Part model, mm, in its own coordinate system. A direction names the side the tool comes from. Round coordinates to 2 decimals unless told otherwise and drop trailing zeros. Write each loop counter-clockwise with the first axis right and the second up, starting at its lowest first coordinate (ties: lowest second). Pieces come first, ordered by that corner, then holes.
Autodesk Inventor part; units mm, degrees
ref_plane "YZ Plane" through (0, 0, 0) normal (1, 0, 0) x (0, 1, 0)
ref_plane "XZ Plane" through (0, 0, 0) normal (0, 1, 0) x (-1, 0, 0)
ref_plane "XY Plane" through (0, 0, 0) normal (0, 0, 1) x (1, 0, 0)
sketch "Szkic1" plane through (0, 0, 0) normal (0, 0, 1) x (1, 0, 0)
  line L0 (-10.3866, 5.557) -> (25.6134, 5.557)
  line L1 (25.6134, 5.557) -> (25.6134, -36.443)
  line L2 (25.6134, -36.443) -> (-10.3866, -36.443)
  line L3 (-10.3866, -36.443) -> (-10.3866, 5.557)
  point P0 (0, 0)
  point P1 (20.6134, -0.193)
  point P2 (20.6134, -30.693)
  point P3 (-5.3866, -0.193)
  point P4 (-5.3866, -30.693)
  dimension "d0" = 36
  dimension "d1" = 42
  dimension "d2" = 5
  dimension "d3" = 5
  dimension "d4" = 5
  dimension "d5" = 5
  dimension "d6" = 5.75
  dimension "d7" = 5.75
  dimension "d8" = 5.75
  dimension "d9" = 5.75
extrude "Wyciągnięcie proste1" add sketch "Szkic1" along normal blind 7.5
hole "Otwór1" at (20.6134, -0.193, 0) at (20.6134, -30.693, 0) at (-5.3866, -0.193, 0) at (-5.3866, -30.693, 0) direction (0, 0, 1) diameter 5 end through all
sketch "Szkic2" plane through (-10.3866, -36.443, 0) normal (0, -1, 0) x (1, 0, 0)
  line L0 (36, 0) -> (0, 0)
  line L1 (36, 0) -> (36, 7.5)
  line L2 (0, 7.5) -> (36, 7.5)
  line L3 (0, 0) -> (0, 7.5)
  line L4 (36, 7.5) -> (0, 7.5)
  circle A0 centre (18, 8.5) radius 5.05
  point P0 (10.3866, 0)
  dimension "d19" = 36
  dimension "d25" = 8.5
  dimension "d26" = 18
  dimension "d27" = 10.1
extrude "Wyciągnięcie proste2" cut sketch "Szkic2" against normal through all contours A0 L2 | L2 A0
sketch "Szkic3" plane through (0, 0, 7.5) normal (0, 0, 1) x (1, 0, 0)
  line L0 (25.6134, 5.557) -> (12.5634, 5.557)
  line L1 (12.5634, 5.557) -> (12.5634, -36.443)
  line L2 (-10.3866, -36.443) -> (2.6634, -36.443)
  line L3 (25.6134, -36.443) -> (25.6134, 5.557)
  circle A0 centre (20.6134, -0.193) radius 2.5
  circle A1 centre (20.6134, -30.693) radius 2.5
  line L4 (12.5634, -36.443) -> (25.6134, -36.443)
  line L5 (2.6634, -36.443) -> (2.6634, 5.557)
  line L6 (2.6634, 5.557) -> (-10.3866, 5.557)
  line L7 (-10.3866, 5.557) -> (-10.3866, -36.443)
  point P0 (0, 0)
extrude "Wyciągnięcie proste3" add sketch "Szkic3" along normal blind 1 contours L3 L4 L1 L0
sketch "Szkic4" plane through (0, 0, 0) normal (0, 0, -1) x (-1, 0, 0)
  circle A0 centre (5.3866, -0.193) radius 2.5
  circle A1 centre (-20.6134, -0.193) radius 2.5
  circle A2 centre (-20.6134, -30.693) radius 2.5
  circle A3 centre (5.3866, -30.693) radius 2.5
  line L0 (10.3866, 5.557) -> (-25.6134, 5.557)
  line L1 (-25.6134, 5.557) -> (-25.6134, -36.443)
  line L2 (-25.6134, -36.443) -> (10.3866, -36.443)
  line L3 (10.3866, -36.443) -> (10.3866, 5.557)
  line L4 (-25.6134, 5.557) -> (-25.6134, 23.557)
  line L5 (-25.6134, 23.557) -> (-19.6134, 23.557)
  line L6 (-19.6134, 23.557) -> (-19.6134, 5.557)
  point P0 (0, 0)
  dimension "d30" = 18
  dimension "d31" = 6
extrude "Wyciągnięcie proste4" add sketch "Szkic4" against normal blind 8.5 contours L0 L4 L5 L6
sketch "Szkic5" plane through (19.6134, 5.557, 0) normal (-1, 0, 0) x (0, 0, 1)
  line L0 (0, 0) -> (0, 18)
  line L1 (8.5, 0) -> (0, 0)
  line L2 (8.5, 18) -> (8.5, 0)
  line L3 (0, 18) -> (8.5, 18)
  point P0 (0, -5.557)
  point P1 (4.25, 14)
  dimension "d34" = 4.25
  dimension "d35" = 4
  dimension "d47" = 8.5
hole "Otwór2" at (19.6134, 19.557, 4.25) direction (1, 0, 0) diameter 3 end through all
chamfer "Faza1" distance 3 angle 45 1 edges at (19.6134, 5.557, 4.25)
fillet "Zaokrąglenie2" radius 1 5 edges at (-10.3866, 5.557, 3.75) (-10.3866, -36.443, 3.75) (25.6134, -36.443, 4.25) (19.6134, 8.557, 4.25) (16.6134, 5.557, 4.25)
sketch "Szkic6" plane through (7.6134, -36.443, 8.5) normal (0, -1, 0) x (1, 0, 0)
  line L0 (17, 0) -> (17, -8.5)
  line L1 (4.95, 0) -> (17, 0)
  line L2 (4.95, -1) -> (4.95, 0)
  arc A0 (-4.95, -1) -> (4.95, -1) centre (0, 0) ccw
  line L3 (-17, -1) -> (-4.95, -1)
  line L4 (-17, -8.5) -> (-17, -1)
  line L5 (17, -8.5) -> (-17, -8.5)
  circle A1 centre (0, 0) radius 5.05
  point P0 (-7.6134, -8.5)
  dimension "d49" = 10.1
extrude "Wyciągnięcie proste5" cut sketch "Szkic6" against normal through all contours A1 L2 L1 | L1 L2 A0 A1
fillet "Zaokrąglenie3" radius 0.5 2 edges at (19.6134, 23.557, 4.25) (25.6134, 23.557, 4.25)
properties part number "3DP_ABS_X_Axis_Linear_Shaft_Clamp_Bottom_With_Endstop_Screw"
Q1. Cut at B-B on y = -29.5. Write the cut outline in (x, z).
Values follow:
outline: (-10.39, 0) - (-7.58, 0) - (-7.58, 7.5) - (-10.39, 7.5) - close; (-3.19, 0) - (18.42, 0) - (18.42, 8.5) - (12.66, 8.5) arc R5.05 cw to (2.66, 7.5) - (-3.19, 7.5) - close; (22.81, 0) - (25.61, 0) - (25.61, 8.5) - (22.81, 8.5) - close
Q2. Drop flat-ended pins along their axis: pin 1 (2.5 mm diameter, centred on y = 14.5, z = 3.5, fed in from -X); pin 2 (4 mm diameter, centred on x = 2, z = 6, fed in from +Y); pin 3 (6.5 mm diameter, centred on x = -4.5, y = -8.5, fed in from +Z). Give the stop position or say it passes through.
Values follow:
pin 1: stops at x = 19.61
pin 2: stops at y = 5.56
pin 3: stops at z = 7.5
Q3. Cut at D-D on z = 1. Write the cut outline in (x, y).
Values follow:
outline: (-10.39, -35.44) arc R1 ccw to (-9.39, -36.44) - (24.61, -36.44) arc R1 ccw to (25.61, -35.44) - (25.61, 23.06) arc R0.5 ccw to (25.11, 23.56) - (20.11, 23.56) arc R0.5 ccw to (19.61, 23.06) - (19.61, 8.97) arc R1 cw to (19.32, 8.26) - (16.91, 5.85) arc R1 cw to (16.2, 5.56) - (-9.39, 5.56) arc R1 ccw to (-10.39, 4.56) - close; hole circle Ø5 at (-5.39, -30.69); hole circle Ø5 at (-5.39, -0.19); hole circle Ø5 at (20.61, -30.69); hole circle Ø5 at (20.61, -0.19)
Q4. Cut at C-C on x = -7. Write the cut outline in (y, z).
Values follow:
outline: (-36.44, 0) - (-32.6, 0) - (-32.6, 7.5) - (-36.44, 7.5) - close; (-28.78, 0) - (-2.1, 0) - (-2.1, 7.5) - (-28.78, 7.5) - close; (1.72, 0) - (5.56, 0) - (5.56, 7.5) - (1.72, 7.5) - close
Q5. Mould opens along X. For faces 3 (the cylindrical face through (-3.87, -32.68, 3.8)), 4 (the flat face through (-4, -15, 7.5)), 5 (the flat face through (18.097, 7.04, 4.19)) say: +X half, -X half, draft (parallel to the pull), parting line (faces both ways), or undercut.
Values follow:
face 3: undercut
face 4: draft
face 5: -X half
Q6. Wall check: L1, parallel to X at y = 0, z = 0.5; L2, parallel to Y at x = 20, z = 0.5; L3, parallel to Y at x = -4, z = 4.25. Give the ranges that are in metal, low to high.
Values follow:
L1: x = -10.39 to -7.88, -2.89 to 18.12, 23.11 to 25.61
L2: y = -36.44 to -33.12, -28.27 to -2.62, 2.23 to 23.54
L3: y = -36.44 to -32.77, -28.61 to -2.27, 1.89 to 5.56
Q7. Cut at A-A on z = 4.25. Write the cut outline in (x, y), plus the area to 3 significant figures.
Values follow:
outline: (-10.39, -35.44) arc R1 ccw to (-9.39, -36.44) - (4.89, -36.44) - (4.89, 5.56) - (-9.39, 5.56) arc R1 ccw to (-10.39, 4.56) - close; (10.34, -36.44) - (24.61, -36.44) arc R1 ccw to (25.61, -35.44) - (25.61, 18.06) - (19.61, 18.06) - (19.61, 8.97) arc R1 cw to (19.32, 8.26) - (16.91, 5.85) arc R1 cw to (16.2, 5.56) - (10.34, 5.56) - close; (19.61, 21.06) - (25.61, 21.06) - (25.61, 23.06) arc R0.5 ccw to (25.11, 23.56) - (20.11, 23.56) arc R0.5 ccw to (19.61, 23.06) - close; hole circle Ø5 at (-5.39, -30.69); hole circle Ø5 at (-5.39, -0.19); hole circle Ø5 at (20.61, -30.69); hole circle Ø5 at (20.61, -0.19)
area: 1,300 mm2
Q8. Which spindle directions (+Z, -Z, +X, -X, +Y, -Y) get a long thin tool onto all of the face, cutting with end or side? Do faces 1 (the flat face through (4, 5.557, 3)), 2 (the cylindrical face through (-2.946, -0.735, 3.802)). Say none if no direction does.
Values follow:
face 1: +Z, -Z, -X, +Y
face 2: +Z, -Z
